from build123d import *

# Parameters (mm, degrees)
F0_R     = 26.2001
F0_R_2   = 1.778
F0_R_3   = 6.35
F1_DEPTH = 6.35


with BuildPart() as f1:
    # F0 (on Front) → F1 (new body)
    with BuildSketch(Plane.XZ):
        Circle(F0_R)
        with Locations((-13.470384, -13.470384)):
            Circle(F0_R_2, mode=Mode.SUBTRACT)
        with Locations((-7.290119, -17.599905)):
            Circle(F0_R_2, mode=Mode.SUBTRACT)
        with Locations((0, -19.05)):
            Circle(F0_R_2, mode=Mode.SUBTRACT)
        with Locations((-17.599905, -7.290119)):
            Circle(F0_R_2, mode=Mode.SUBTRACT)
        with Locations((-19.05, 0)):
            Circle(F0_R_2, mode=Mode.SUBTRACT)
        with Locations((-6.914797, -6.914797)):
            Circle(F0_R_2, mode=Mode.SUBTRACT)
        with Locations((0, -9.779)):
            Circle(F0_R_2, mode=Mode.SUBTRACT)
        with Locations((-9.779, 0)):
            Circle(F0_R_2, mode=Mode.SUBTRACT)
        Circle(F0_R_3, mode=Mode.SUBTRACT)
        with Locations((7.290119, -17.599905)):
            Circle(F0_R_2, mode=Mode.SUBTRACT)
        with Locations((13.470384, -13.470384)):
            Circle(F0_R_2, mode=Mode.SUBTRACT)
        with Locations((6.914797, -6.914797)):
            Circle(F0_R_2, mode=Mode.SUBTRACT)
        with Locations((9.779, 0)):
            Circle(F0_R_2, mode=Mode.SUBTRACT)
        with Locations((17.599905, -7.290119)):
            Circle(F0_R_2, mode=Mode.SUBTRACT)
        with Locations((19.05, 0)):
            Circle(F0_R_2, mode=Mode.SUBTRACT)
        with Locations((-17.599905, 7.290119)):
            Circle(F0_R_2, mode=Mode.SUBTRACT)
        with Locations((-6.914797, 6.914797)):
            Circle(F0_R_2, mode=Mode.SUBTRACT)
        with Locations((0, 9.779)):
            Circle(F0_R_2, mode=Mode.SUBTRACT)
        with Locations((-13.470384, 13.470384)):
            Circle(F0_R_2, mode=Mode.SUBTRACT)
        with Locations((-7.290119, 17.599905)):
            Circle(F0_R_2, mode=Mode.SUBTRACT)
        with Locations((0, 19.05)):
            Circle(F0_R_2, mode=Mode.SUBTRACT)
        with Locations((6.914797, 6.914797)):
            Circle(F0_R_2, mode=Mode.SUBTRACT)
        with Locations((17.599905, 7.290119)):
            Circle(F0_R_2, mode=Mode.SUBTRACT)
        with Locations((7.290119, 17.599905)):
            Circle(F0_R_2, mode=Mode.SUBTRACT)
        with Locations((13.470384, 13.470384)):
            Circle(F0_R_2, mode=Mode.SUBTRACT)
    extrude(amount=F1_DEPTH)


solid = f1.part
Check sheet for the modelled part. Datum: model origin and axes. Units: mm. Coordinates: 2 decimals unless noted, no trailing zeros. Loops run counter-clockwise (first coordinate to the right, second up) from the corner with the lowest first, then second, coordinate; pieces in that order, holes last. Notation, with made-up numbers: (34, -32) -> (63, -32) arc R36 cw to (63, 7) -> close; hole circle Ø6 at (21.25, 33.25). An arc over 180 degrees is marked (long way). Write item = value, one per line. Start each with the question number.
1. Section check C-C on y = -2. Give the number of separate pieces and of enclosed holes in the cut face, then the cut area to 3 significant figures.
2. Section check D-D on x = 13. Record the cut outline in (y, z), then the cut area to 3 significant figures.
3. Section check A-A on x = 0. Record the cut outline in (y, z), then the cut area to 3 significant figures.
4. Depth check by flat-ended pin: P1, Ø5.5, axis at x = -17.6, z = -7.29, coming from the -Y side; P2, Ø1.5, axis at y = -2.5, z = -18, coming from the +X side; P3, Ø1.5, axis at x = -20, y = -1.5, coming from the +Z side. Enter the tip coordinate at first touch or a pass-through.
5. Section check B-B on z = 0. Record the cut outline in (x, y).
6. Material ranges on line 1 (Z direction, x = 19.05, y = -2.75); line 2 (Z direction, x = 0, y = -3); line 3 (X direction, y = -3.25, z = -14.5), recorded low to high.
7. Draft check along X on faces 1 (the cylindrical face through (7.059, -3.131, -15.837)), 2 (the flat face through (5, -6.35, -5)). Enter one of: released by +X, released by -X, zero draft, split by the parting line, or undercut.
Responses:
q1.separate_pieces = 1
q1.enclosed_holes = 25
q1.area = 1,790 mm2
q2.outline = (-6.35, -22.75) -> (0, -22.75) -> (0, -15.19) -> (-6.35, -15.19) -> close; (-6.35, -11.76) -> (0, -11.76) -> (0, 11.76) -> (-6.35, 11.76) -> close; (-6.35, 15.19) -> (0, 15.19) -> (0, 22.75) -> (-6.35, 22.75) -> close
q2.area = 245 mm2
q3.outline = (-6.35, -26.2) -> (0, -26.2) -> (0, -20.83) -> (-6.35, -20.83) -> close; (-6.35, -17.27) -> (0, -17.27) -> (0, -11.56) -> (-6.35, -11.56) -> close; (-6.35, -8) -> (0, -8) -> (0, -6.35) -> (-6.35, -6.35) -> close; (-6.35, 6.35) -> (0, 6.35) -> (0, 8) -> (-6.35, 8) -> close; (-6.35, 11.56) -> (0, 11.56) -> (0, 17.27) -> (-6.35, 17.27) -> close; (-6.35, 20.83) -> (0, 20.83) -> (0, 26.2) -> (-6.35, 26.2) -> close
q3.area = 162 mm2
q4.P1 = -6.35
q4.P2 = 19.72
q4.P3 = 17.77
q5.outline = (-26.2, -6.35) -> (-20.83, -6.35) -> (-20.83, 0) -> (-26.2, 0) -> close; (-17.27, -6.35) -> (-11.56, -6.35) -> (-11.56, 0) -> (-17.27, 0) -> close; (-8, -6.35) -> (-6.35, -6.35) -> (-6.35, 0) -> (-8, 0) -> close; (6.35, -6.35) -> (8, -6.35) -> (8, 0) -> (6.35, 0) -> close; (11.56, -6.35) -> (17.27, -6.35) -> (17.27, 0) -> (11.56, 0) -> close; (20.83, -6.35) -> (26.2, -6.35) -> (26.2, 0) -> (20.83, 0) -> close
q6.line_1 = -17.99 to -8.32, -6.26 to -1.78, 1.78 to 6.26, 8.32 to 17.99
q6.line_2 = -26.2 to -20.83, -17.27 to -11.56, -8 to -6.35, 6.35 to 8, 11.56 to 17.27, 20.83 to 26.2
q6.line_3 = -21.82 to -14.92, -12.02 to 12.02, 14.92 to 21.82
q7.face_1 = undercut
q7.face_2 = zero draft
